```python
from build123d import *

# Parameters (mm, degrees)
F1_DEPTH = 10


with BuildPart() as f1:
    # F0 (on Top) → F1 (new body)
    with BuildSketch(Plane.XY):
        with BuildLine():
            ThreePointArc((0, 380), (5, 385), (0, 390))
            ThreePointArc((0, 390), (-200.003129, 210.088535), (-42.190413, -7.775031))
            ThreePointArc((-42.190413, -7.775031), (-31.760642, -9.442202), (-21.213203, -10))
            Line((-21.213203, -10), (0, -10))
            Line((0, -10), (12.941731, -10))
            ThreePointArc((12.941731, -10), (33.571927, -12.151162), (53.314545, -18.5121))
            ThreePointArc((53.314545, -18.5121), (164.293465, -219.555515), (0, -380))
            ThreePointArc((0, -380), (-5, -385), (0, -390))
            ThreePointArc((0, -390), (200.003129, -210.088535), (42.190413, 7.775031))
            ThreePointArc((42.190413, 7.775031), (31.760642, 9.442202), (21.213203, 10))
            Line((21.213203, 10), (0, 10))
            Line((0, 10), (-12.941731, 10))
            ThreePointArc((-12.941731, 10), (-33.571927, 12.151162), (-53.314545, 18.5121))
            ThreePointArc((-53.314545, 18.5121), (-164.293465, 219.555515), (0, 380))
        make_face()
    extrude(amount=F1_DEPTH)


solid = f1.part
```
Verification items for the finished model (mm, model axes). Give positions to 0.01 mm unless a question says otherwise; leave off trailing zeros. Order: outer loops, then holes, each group sorted by start corner. A loop starts at its lowest first (then second) coordinate and runs counter-clockwise, first axis right, second up. Notation, with made-up numbers: M 68,40 L 120,40 A7 ccw 120,46 Z; hole C 1,34.25 d2. An arc over 180 degrees is marked long. Return JSON: item names as keys, results as strings. Group by question number.
1) Section check B-B on x = -146.5. Record the cut outline in (y, z).
2) Mould release check, pull along Y, two halves, no side actions. Record for faces 1 (the face through (-1, 2, 10)), 2 (the face through (-164.766, 216.134, 4.93)), 3 (the face through (-199.526, 214.186, 4.93)): pulls with the +Y half, pulls with the -Y half, needs draft (parallel to the pull), parting line crosses it, or undercut.
3) Section check A-A on z = 4.75. Record the cut outline in (x, y) (3 decimals), and give its area (3 significant figures).
4) Section check C-C on y = 250.5. Record the cut outline in (x, z).
5) Section check D-D on y = -197.5. Record the cut outline in (x, z).
6) Go/stop test with flat-tipped pins: pin 1 Ø3 at (x, z) = (-3, 4) entering from -Y; pin 2 Ø5 at (x, z) = (61.5, 8) entering from +Y; pin 3 Ø6 at (y, z) = (92.5, 8.5) entering from +X. Record where each tip stops, or that it passes through.
7) Scan lines: line 1 (Y direction, x = 152, z = 7); line 2 (Y direction, x = 116.5, z = 6.25); line 3 (X direction, y = -337, z = 8.5). Record each from-to range of solid material in increasing order.
Answer block:
{
 "1": {"outline": "M 51.07,0 L 107.52,0 L 107.52,10 L 51.07,10 Z; M 276.29,0 L 326.68,0 L 326.68,10 L 276.29,10 Z"},
 "2": {"face 1": "needs draft", "face 2": "undercut", "face 3": "parting line crosses it"},
 "3": {"outline": "M -53.315,18.512 A189.523 cw 0,380 A5 ccw 0,390 A201.125 ccw -42.19,-7.775 A100 ccw -21.213,-10 L 12.942,-10 A100 cw 53.315,-18.512 A189.523 cw 0,-380 A5 ccw 0,-390 A201.125 ccw 42.19,7.775 A100 ccw 21.213,10 L -12.942,10 A100 cw Z", "area": "32,000 mm^2"},
 "4": {"outline": "M -191.45,0 L -157.04,0 L -157.04,10 L -191.45,10 Z"},
 "5": {"outline": "M 166.24,0 L 200.94,0 L 200.94,10 L 166.24,10 Z"},
 "6": {"pin 1": "stops at y = -389.77", "pin 2": "stops at y = 3.4", "pin 3": "stops at x = -136.27"},
 "7": {"line 1": "y = -320.58 to -264.18, -119.63 to -57.17", "line 2": "y = -352.82 to -319.97, -63.83 to -24.93", "line 3": "x = 98.72 to 136.05"}
}
